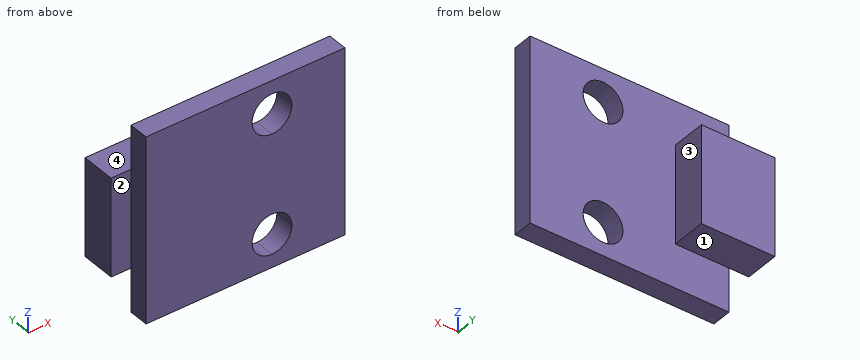
```python
from build123d import *

# Parameters (mm, degrees)
SKETCH_1_W      = 3
SKETCH_1_H      = 14
SKETCH_1_W_2    = 4.05
SKETCH_1_H_2    = 7.4
EXTRUDE_1_DEPTH = 1.5
EXTRUDE_START   = 1.5
SKETCH_1_3_W    = 5.55
SKETCH_1_3_H    = 7.4
EXTRUDE_2_DEPTH = 2.6


with BuildPart() as part:
    # Эскиз1 → Бобышка-Вытянуть1 (new body)
    with BuildSketch(Plane(origin=(0, 0, 0), x_dir=(1, 0, 0), z_dir=(0, 1, 0))):
        with BuildLine():
            Line((4.5, 7), (2, 7))
            Line((2, 7), (2, 6))
            ThreePointArc((2, 6), (3.060660172, 5.560660172), (3.5, 4.5))
            ThreePointArc((3.5, 4.5), (3.060660172, 3.439339828), (2, 3))
            Line((2, 3), (2, -3))
            ThreePointArc((2, -3), (3.060660172, -3.439339828), (3.5, -4.5))
            ThreePointArc((3.5, -4.5), (3.060660172, -5.560660172), (2, -6))
            Line((2, -6), (2, -7))
            Line((2, -7), (4.5, -7))
            Line((4.5, -7), (4.5, 7))
        make_face()
        with Locations((6, 0)):
            Rectangle(SKETCH_1_W, SKETCH_1_H)
        with BuildLine():
            Line((-7.5, 7), (-7.5, 3.7))
            Line((-7.5, 3.7), (-3.45, 3.7))
            Line((-3.45, 3.7), (-3.45, -3.7))
            Line((-3.45, -3.7), (-7.5, -3.7))
            Line((-7.5, -3.7), (-7.5, -7))
            Line((-7.5, -7), (2, -7))
            Line((2, -7), (2, -6))
            ThreePointArc((2, -6), (0.5, -4.5), (2, -3))
            Line((2, -3), (2, 3))
            ThreePointArc((2, 3), (0.5, 4.5), (2, 6))
            Line((2, 6), (2, 7))
            Line((2, 7), (-7.5, 7))
        make_face()
        with Locations((-5.475, 0)):
            Rectangle(SKETCH_1_W_2, SKETCH_1_H_2)
    extrude(amount=EXTRUDE_1_DEPTH)

    # Эскиз1<3> → Бобышка-Вытянуть2 (add)
    with BuildSketch(Plane(origin=(0, 0, 0), x_dir=(1, 0, 0), z_dir=(0, 1, 0)).offset(EXTRUDE_START)):
        with Locations((-6.225, 0)):
            Rectangle(SKETCH_1_3_W, SKETCH_1_3_H)
    extrude(amount=EXTRUDE_2_DEPTH)


solid = part.part
```
CAD build for the part. Positions are in the model's coordinates, mm. Face numbers are marked on the shaded views. A direction names the side the tool comes from. Coordinates: 2 decimals unless noted, no trailing zeros. Write each loop counter-clockwise with the first axis right and the second up, starting at its lowest first coordinate (ties: lowest second). Pieces come first, ordered by that corner, then holes. Notation, with made-up numbers: (28.5, 0) -> (51.5, 0) arc R21 ccw to (51.5, 26) -> close; hole circle Ø8 at (49.25, 18). An arc over 180 degrees is marked (long way). Use CSV: the item, a comma, the result in double quotes. Start each with the question number.
Item 1: Drop flat-ended pins along their axis: P1, Ø1.3, axis at y = 3, z = -0.5, coming from the +X side; P2, Ø2, axis at x = -6.5, y = 3, coming from the -Z side; P3, Ø0.8, axis at y = 0.5, z = 1, coming from the -X side. Give the stop position or say it passes through.
Item 2: Band-saw the part on C-C, the plane z = 1.25. Write the cut outline in (x, y).
Item 3: Tool access for the marked faces 1, 2, 3 and 4: list every direction of +Z, -Z, +X, -X, +Y, -Y with a clear straight run to the whole face (end or side of a thin tool).
Item 4: Wall check: probe 1 along Y at (x, z) = (-4, 6.25); probe 2 along X at (y, z) = (1.75, 1.25); probe 3 along Z at (x, y) = (-5.25, 2). Give the ranges that are in metal, low to high.
Item 5: Band-saw the part on B-B, the plane x = -5.5. Write the cut outline in (y, z).
Item 6: Band-saw the part on D-D, the plane x = 3.25. Write the cut outline in (y, z), plus the area to 3 significant figures.
Item 7: Band-saw the part on A-A, the plane y = 1.3. Write the cut outline in (x, z), plus the area to 3 significant figures.
Response values:
1,P1,"stops at x = -3.45"
1,P2,"stops at z = -3.7"
1,P3,"stops at x = -7.5"
2,outline,"(-9, 1.5) -> (-7.5, 1.5) -> (-7.5, 0) -> (7.5, 0) -> (7.5, 1.5) -> (-3.45, 1.5) -> (-3.45, 4.1) -> (-9, 4.1) -> close"
3,face 1,"-Z, +X, -X, +Y"
3,face 2,"+Z, -Z, -X, -Y"
3,face 3,"+Z, -Z, +X, +Y"
3,face 4,"+Z, +X, -X, +Y"
4,probe 1,"y = 0 to 1.5"
4,probe 2,"x = -9 to -3.45"
4,probe 3,"z = -3.7 to 3.7"
5,outline,"(0, -7) -> (1.5, -7) -> (1.5, -3.7) -> (4.1, -3.7) -> (4.1, 3.7) -> (1.5, 3.7) -> (1.5, 7) -> (0, 7) -> close"
6,outline,"(0, -7) -> (1.5, -7) -> (1.5, -5.33) -> (0, -5.33) -> close; (0, -3.67) -> (1.5, -3.67) -> (1.5, 3.67) -> (0, 3.67) -> close; (0, 5.33) -> (1.5, 5.33) -> (1.5, 7) -> (0, 7) -> close"
6,area,"16.0 mm2"
7,outline,"(-7.5, -7) -> (7.5, -7) -> (7.5, 7) -> (-7.5, 7) -> close; hole circle Ø3 at (2, -4.5); hole circle Ø3 at (2, 4.5)"
7,area,"196 mm2"
